Input: part model. Units: mm. Frame: model coordinates. A direction names the side the tool comes from. Coordinates: 2 decimals unless noted, no trailing zeros. Loops run counter-clockwise (first coordinate to the right, second up) from the corner with the lowest first, then second, coordinate; pieces in that order, holes last.
(1) Section D-D, the plane y = 89.5. Return loops of the section in (x, z).
(2) Mould query, pull axis Y, two halves, no side actions, for faces 1 (the face through (-1, 12, 8)), 2 (the face through (-35.567, 6.563, 4.056)), 3 (the face through (26, 122.23, 4)). Classes: released by +Y, released by -Y, zero draft, split by the parting line, or undercut.
(3) Section B-B, the plane x = -36. Return loops of the section in (y, z), then the cut area to 3 significant figures.
(4) Contact query for flat-ended pins moving along their axis: P1, Ø1.5, axis at y = -32, z = 1.5, coming from the +X side; P2, Ø1, axis at x = 43, z = 4.5, coming from the -Y side; P3, Ø4, axis at x = 37.5, z = 3, coming from the -Y side. Output: stop coordinate, or through.
(5) Line query: L1, parallel to X at y = 107, z = 6.75; L2, parallel to Y at x = 10, z = 5.25; L3, parallel to Y at x = -31.5, z = 6. Output: solid intervals per line, ascending.
(6) Section A-A, the plane z = 1.25. Return loops of the section in (x, y), then the cut area to 3 significant figures.
(7) Set-up query: faces 4 (the face through (23.53, 103, 4)), 5 (the face through (29.53, 88, 4)), 6 (the face through (0, -38.126, 4)). Return all of +Z, -Z, +X, -X, +Y, -Y with unobstructed straight access to the full face (end or side cutting, diameter ignored); none if empty.
(8) Section C-C, the plane x = 0. Return loops of the section in (y, z), then the cut area to 3 significant figures.
```python
from build123d import *

# Parameters (mm, degrees)
PAD_DEPTH          = 8
SKETCH001_W        = 24.2
SKETCH001_H        = 8.2
POCKET_DEPTH       = 8
POLARPATTERN_COUNT = 3


with BuildPart() as part:
    # Sketch → Pad (new body)
    with BuildSketch(Plane.XY):
        with BuildLine():
            ThreePointArc((-29.53026, 52.229912), (0, -60), (29.53026, 52.229912))
            Line((29.53026, 122.229912), (29.53026, 52.229912))
            Line((23.53026, 122.229912), (29.53026, 122.229912))
            Line((23.53026, 122.229912), (23.53026, 82.229912))
            Line((23.53026, 82.229912), (-29.53026, 52.229912))
        make_face()
    extrude(amount=PAD_DEPTH)

    # Sketch001 → Pocket (cut)
    with BuildSketch(Plane.XY.offset(8)):
        with Locations((0, -34.025975)):
            Rectangle(SKETCH001_W, SKETCH001_H)
    pocket = extrude(amount=-POCKET_DEPTH, mode=Mode.SUBTRACT)

    # PolarPattern: Pocket ×3 about axis
    polarpattern_axis = Axis((0, 0, 8), (0, 0, 1))
    for i in range(1, POLARPATTERN_COUNT):
        add(pocket.rotate(polarpattern_axis, i * 360 / POLARPATTERN_COUNT), mode=Mode.SUBTRACT)


solid = part.part
```
Report:
1. outline: (23.53, 0) - (29.53, 0) - (29.53, 8) - (23.53, 8) - close
2. face 1: zero draft
2. face 2: undercut
2. face 3: released by +Y
3. outline: (-48, 0) - (6.81, 0) - (6.81, 8) - (-48, 8) - close; (13.9, 0) - (48, 0) - (48, 8) - (13.9, 8) - close
3. area: 711 mm2
4. P1: stops at x = 51.22
4. P2: stops at y = -42.35
4. P3: stops at y = -48.37
5. L1: x = 23.53 to 29.53
5. L2: y = -59.16 to -38.13, -29.93 to 74.58
5. L3: y = -51.07 to 5.29, 21.69 to 51.07
6. outline: (-29.53, 52.23) arc R60 ccw (long way) to (29.53, 52.23) - (29.53, 122.23) - (23.53, 122.23) - (23.53, 82.23) - close; hole (-39.07, 8.58) - (-31.97, 4.48) - (-19.87, 25.44) - (-26.97, 29.54) - close; hole (-12.1, -38.13) - (12.1, -38.13) - (12.1, -29.93) - (-12.1, -29.93) - close; hole (19.87, 25.44) - (31.97, 4.48) - (39.07, 8.58) - (26.97, 29.54) - close
6. area: 11,600 mm2
7. face 4: +Z, -Z, -X, +Y
7. face 5: +Z, -Z, +X, +Y
7. face 6: +Z, -Z
8. outline: (-60, 0) - (-38.13, 0) - (-38.13, 8) - (-60, 8) - close; (-29.93, 0) - (68.93, 0) - (68.93, 8) - (-29.93, 8) - close
8. area: 966 mm2
